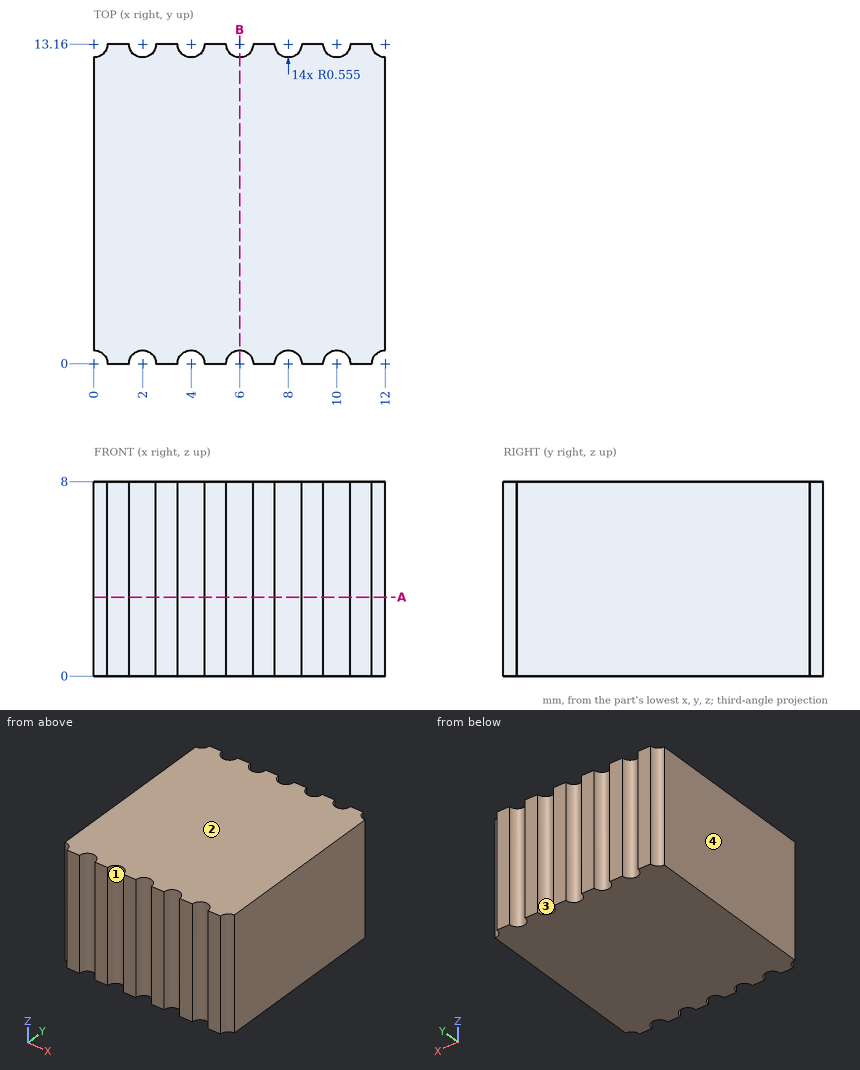
Part print with two shaded views. Sizes in mm from the minimum x, y, z corner. Coordinates: 2 decimals unless noted, no trailing zeros. Order: outer loops, then holes, each group sorted by start corner. A loop starts at its lowest first (then second) coordinate and runs counter-clockwise, first axis right, second up. Notation, with made-up numbers: (56, 15) - (96, 15) arc R36 ccw to (96, 49) - close; hole circle Ø10 at (57, 60.5). An arc over 180 degrees is marked (long way). Write item = value, one per line. Start each with the question number.
1) Two-plate mould, pull along X, no slides. Class the marked faces 1, 2, 3 and 4: pulls with the +X half, pulls with the -X half, needs draft (parallel to the pull), parting line crosses it, or undercut.
2) Saw through at B-B on x = 6. Write the cut outline in (y, z) (3 decimals).
3) Saw through at A-A on z = 3.25. Write the cut outline in (x, y) (3 decimals).
4) Wall check: line 1 along Y through (x, z) = (8, 1.75) (3 decimals). Give the ranges that are in metal, low to high. Write a range as from..to.
From the geometry:
q1.face_1 = undercut
q1.face_2 = needs draft
q1.face_3 = undercut
q1.face_4 = pulls with the -X half
q2.outline = (0.555, 0) - (12.605, 0) - (12.605, 8) - (0.555, 8) - close
q3.outline = (0, 0.555) arc R0.555 cw to (0.555, 0) - (1.445, 0) arc R0.555 cw to (2.555, 0) - (3.445, 0) arc R0.555 cw to (4.555, 0) - (5.445, 0) arc R0.555 cw to (6.555, 0) - (7.445, 0) arc R0.555 cw to (8.555, 0) - (9.445, 0) arc R0.555 cw to (10.555, 0) - (11.445, 0) arc R0.555 cw to (12, 0.555) - (12, 12.605) arc R0.555 cw to (11.445, 13.16) - (10.555, 13.16) arc R0.555 cw to (9.445, 13.16) - (8.555, 13.16) arc R0.555 cw to (7.445, 13.16) - (6.555, 13.16) arc R0.555 cw to (5.445, 13.16) - (4.555, 13.16) arc R0.555 cw to (3.445, 13.16) - (2.555, 13.16) arc R0.555 cw to (1.445, 13.16) - (0.555, 13.16) arc R0.555 cw to (0, 12.605) - close
q4.line_1 = 0.555..12.605
